Check sheet for the drawn part. Datum: minimum x, y, z corner. Units: mm. Give positions to 0.01 mm unless a question says otherwise; leave off trailing zeros. Write each loop counter-clockwise with the first axis right and the second up, starting at its lowest first coordinate (ties: lowest second). Pieces come first, ordered by that corner, then holes. Notation, with made-up numbers: M -32,45.25 L 19,45.25 A11 ccw 19,64.25 Z; hole C 62,13.5 d5. An arc over 180 degrees is marked long. Write item = value, one per line.
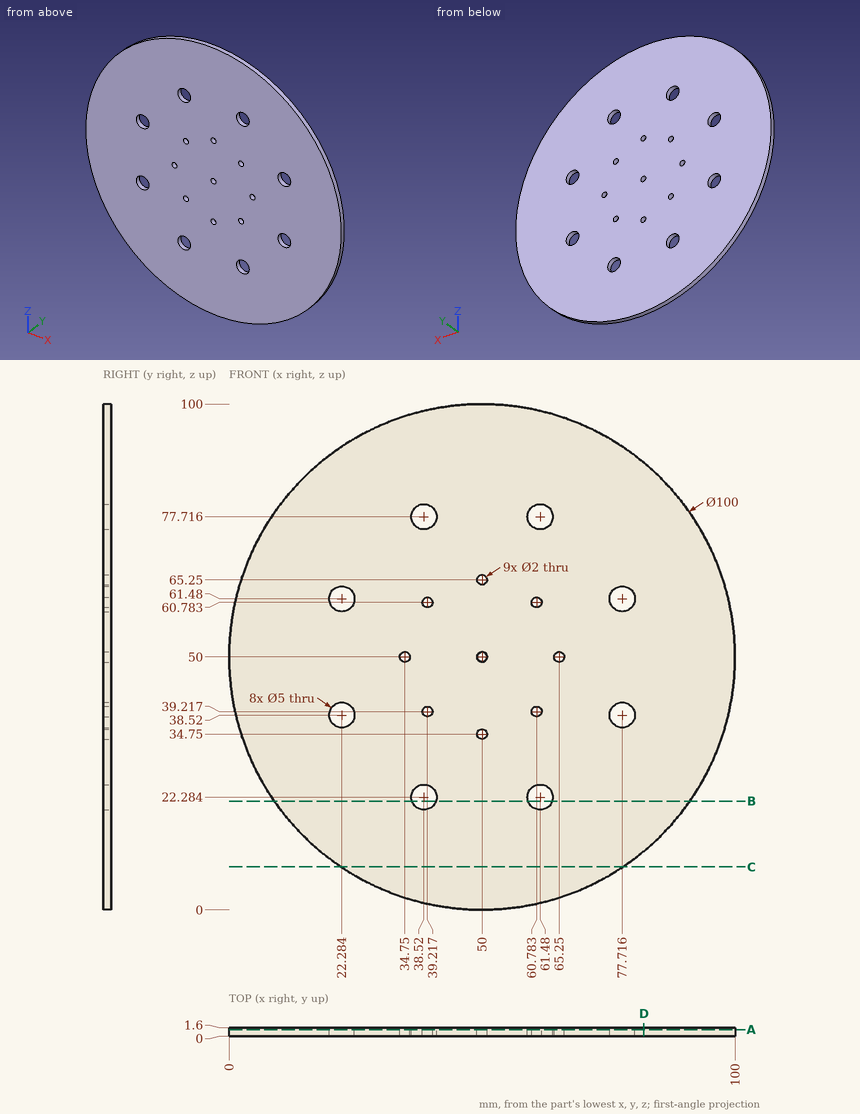
1) Material ranges on probe 1 along Z at (x, y) = (50, 0.65); probe 2 along X at (y, z) = (1.15, 22) (1 decimal), recorded low to high. Write a range as from..to.
From the geometry:
probe_1 = 0..33.75, 35.75..49, 51..64.25, 66.25..100
probe_2 = 8.6..36, 41..59, 64..91.4
2) Cross-section at A-A on y = 1.25. Count the separate pieces of the cut face and the enclosed holes in it, plus the area to 3 significant figures.
From the geometry:
separate_pieces = 1
enclosed_holes = 17
area = 7,670 mm^2
3) Depth check by flat-ended pin: P1, Ø3, axis at x = 38.52, z = 77.72, coming from the +Y side. Enter the tip coordinate at first touch or a pass-through.
From the geometry:
P1 = through
4) Cross-section at C-C on z = 8.5. Record the boundary of the cut face in (x, y).
From the geometry:
outline = M 22.11,0 L 77.89,0 L 77.89,1.6 L 22.11,1.6 Z
5) Cross-section at B-B on z = 21.5. Record the boundary of the cut face in (x, y) (1 decimal).
From the geometry:
outline = M 8.9,0 L 36.1,0 L 36.1,1.6 L 8.9,1.6 Z; M 40.9,0 L 59.1,0 L 59.1,1.6 L 40.9,1.6 Z; M 63.9,0 L 91.1,0 L 91.1,1.6 L 63.9,1.6 Z
6) Cross-section at D-D on x = 82. Record the boundary of the cut face in (y, z).
From the geometry:
outline = M 0,11.58 L 1.6,11.58 L 1.6,88.42 L 0,88.42 Z
